```python
from build123d import *

# Parameters (mm, degrees)
ESQUISSE1_W             = 10
ESQUISSE1_H             = 50
BOSS_EXTRU_1_DEPTH      = 5
ESQUISSE4_W             = 10
ESQUISSE4_H             = 12
BOSS_EXTRU_2_DEPTH      = 2
ESQUISSE5_W             = 10
ESQUISSE5_H             = 12
BOSS_EXTRU_3_DEPTH      = 2
ESQUISSE7_R             = 1.5
ENL_V_MAT_EXTRU_2_DEPTH = 23.073899885
ESQUISSE8_R             = 1.5
ENL_V_MAT_EXTRU_3_DEPTH = 23.073899885


with BuildPart() as part:
    # Esquisse1 → Boss.-Extru.1 (new body)
    with BuildSketch(Plane.XY):
        with Locations((-18.961277556, 0.799561998)):
            Rectangle(ESQUISSE1_W, ESQUISSE1_H)
    extrude(amount=BOSS_EXTRU_1_DEPTH)

    # Esquisse4 → Boss.-Extru.2 (add)
    with BuildSketch(Plane.XY.offset(5)):
        with Locations((-18.961277556, 19.799561998)):
            Rectangle(ESQUISSE4_W, ESQUISSE4_H)
    extrude(amount=BOSS_EXTRU_2_DEPTH)

    # Esquisse5 → Boss.-Extru.3 (add)
    with BuildSketch(Plane.XY.offset(5)):
        with Locations((-18.961277556, -18.200438002)):
            Rectangle(ESQUISSE5_W, ESQUISSE5_H)
    extrude(amount=BOSS_EXTRU_3_DEPTH)

    # Esquisse7 → Enlèv. mat.-Extru.2 (cut)
    with BuildSketch(Plane.XY.offset(7)):
        with Locations((-18.961277556, -19.700438002)):
            Circle(ESQUISSE7_R)
    extrude(amount=-ENL_V_MAT_EXTRU_2_DEPTH, mode=Mode.SUBTRACT)

    # Esquisse8 → Enlèv. mat.-Extru.3 (cut)
    with BuildSketch(Plane.XY.offset(7)):
        with Locations((-18.961277556, 21.299561998)):
            Circle(ESQUISSE8_R)
    extrude(amount=-ENL_V_MAT_EXTRU_3_DEPTH, mode=Mode.SUBTRACT)


solid = part.part
```
Here's how the part is built. I have some questions about the finished solid (model axes, mm). A direction names the side the tool comes from. Round coordinates to 2 decimals unless told otherwise and drop trailing zeros. Order: outer loops, then holes, each group sorted by start corner. A loop starts at its lowest first (then second) coordinate and runs counter-clockwise, first axis right, second up. Notation, with made-up numbers: (49, -39.5) -> (70, -39.5) arc R28 cw to (70, -6.5) -> close; hole circle Ø4 at (18.5, 34.25). An arc over 180 degrees is marked (long way). Use a Markdown table: item, result. Add a question column.
(1) Suppose I cut it at B-B, the plane z = 6.5. Please give me the cut outline in (x, y), and give its area (3 significant figures).
(2) Suppose I cut it at A-A, the plane x = -22.25. Please give me the cut outline in (y, z), and give its area (3 significant figures).
(3) I need wall thicknesses on line 1 along Y through (x, z) = (-19, 1.5); line 2 along Y through (x, z) = (-20, 1.5); line 3 along Z through (x, y) = (-20.75, 8.5). Which ranges of each line are inside material? Lowest first, please.
(4) For pin 1 Ø1.8 at (x, y) = (-18.96, -19.7) entering from +Z; pin 2 Ø1 at (x, y) = (-23, 16.5) entering from -Z, each with a flat end and sliding along its axis, tell me the tip position at first contact or that it passes through.
(5) For faces 1 (the face through (-19, 13.8, 6)), 2 (the face through (-18.27, 19.97, 3.55)), which set-ups out of +Z, -Z, +X, -X, +Y, -Y let a thin tool reach every point of the face, with its end or its side?
(6) Suppose I cut it at D-D, the plane y = 11. Please give me the cut outline in (x, z).
(7) Suppose I cut it at C-C, the plane x = -19.75. Please give me the cut outline in (y, z).
Verdict:
| question | item | result |
|---|---|---|
| 1 | outline | (-23.96, -24.2) -> (-13.96, -24.2) -> (-13.96, -12.2) -> (-23.96, -12.2) -> close; (-23.96, 13.8) -> (-13.96, 13.8) -> (-13.96, 25.8) -> (-23.96, 25.8) -> close; hole circle Ø3 at (-18.96, -19.7); hole circle Ø3 at (-18.96, 21.3) |
| 1 | area | 226 mm2 |
| 2 | outline | (-24.2, 0) -> (25.8, 0) -> (25.8, 7) -> (13.8, 7) -> (13.8, 5) -> (-12.2, 5) -> (-12.2, 7) -> (-24.2, 7) -> close |
| 2 | area | 298 mm2 |
| 3 | line 1 | -24.2 to -21.2, -18.2 to 19.8, 22.8 to 25.8 |
| 3 | line 2 | -24.2 to -20.78, -18.62 to 20.22, 22.38 to 25.8 |
| 3 | line 3 | 0 to 5 |
| 4 | pin 1 | through |
| 4 | pin 2 | z = 0 |
| 5 | face 1 | +Z, +X, -X |
| 5 | face 2 | +Z, -Z |
| 6 | outline | (-23.96, 0) -> (-13.96, 0) -> (-13.96, 5) -> (-23.96, 5) -> close |
| 7 | outline | (-24.2, 0) -> (-20.98, 0) -> (-20.98, 7) -> (-24.2, 7) -> close; (-18.42, 0) -> (20.02, 0) -> (20.02, 7) -> (13.8, 7) -> (13.8, 5) -> (-12.2, 5) -> (-12.2, 7) -> (-18.42, 7) -> close; (22.58, 0) -> (25.8, 0) -> (25.8, 7) -> (22.58, 7) -> close |
